```python
from build123d import *

# Parameters (mm, degrees)
F0_W      = 63.5
F0_H      = 50.8
F1_DEPTH  = 88.9
F2_W      = 63.5
F2_H      = 38.1
F3_DEPTH  = 63.501
F5_DEPTH  = 12.701
F7_DEPTH  = 3.048
F9_DEPTH  = 25.401
F11_DEPTH = 50.801


with BuildPart() as f1:
    # F0 (on Front) → F1 (new body)
    with BuildSketch(Plane.XZ):
        Rectangle(F0_W, F0_H)
    extrude(amount=F1_DEPTH)

    # F2 (on face) → F3 (cut, through all)
    with BuildSketch(Plane.YZ.offset(31.75)):
        with Locations((-57.15, 6.35)):
            Rectangle(F2_W, F2_H)
    extrude(amount=-F3_DEPTH, mode=Mode.SUBTRACT)

    # F4 (on face) → F5 (cut, through all)
    with BuildSketch(Plane.XY.offset(-12.7)):
        with BuildLine():
            Line((0, -88.9), (9.5206265251, -88.9))
            Line((9.5206265251, -88.9), (9.5206265251, -57.4386097176))
            ThreePointArc((9.5206265251, -57.4386097176), (0.4771367105, -47.6369581332), (-9.5017243728, -56.4845235209))
            Line((-9.5017243728, -56.4845235209), (-9.5017243728, -88.9))
            Line((-9.5017243728, -88.9), (0, -88.9))
        make_face()
    extrude(amount=-F5_DEPTH, mode=Mode.SUBTRACT)

    # F6 (on face) → F7 (join)
    with BuildSketch(Plane.XY.offset(-12.7)):
        with BuildLine():
            Line((15.748, -88.9), (15.748, -57.15))
            ThreePointArc((15.748, -57.15), (0, -41.402), (-15.748, -57.15))
            Line((-15.748, -57.15), (-15.748, -88.9))
            Line((-15.748, -88.9), (-9.5017243728, -88.9))
            Line((-9.5017243728, -88.9), (-9.5017243728, -56.4845235209))
            ThreePointArc((-9.5017243728, -56.4845235209), (0.4771367105, -47.6369581332), (9.5206265251, -57.4386097176))
            Line((9.5206265251, -57.4386097176), (9.5206265251, -88.9))
            Line((9.5206265251, -88.9), (15.748, -88.9))
        make_face()
    extrude(amount=F7_DEPTH)

    # F8 (on face) → F9 (cut, through all)
    with BuildSketch(Plane.XZ.offset(25.4)):
        with BuildLine():
            ThreePointArc((6.3459234426, 12.927498704), (4.4089615121, 17.2698532126), (0, 19.05))
            Line((0, 19.05), (0, 12.7))
            Line((0, 12.7), (-6.35, 12.7))
            Line((-6.35, 12.7), (-6.35, 0))
            ThreePointArc((-6.35, 0), (0, -6.35), (6.35, 0))
            ThreePointArc((6.35, 0), (6.3499999211, 0.001001282), (6.3499996842, 0.002002564))
            Line((6.3499996842, 0.002002564), (6.3459234426, 12.927498704))
        make_face()
        with BuildLine():
            Line((0, 12.7), (0, 19.05))
            ThreePointArc((0, 19.05), (-4.4901280605, 17.1901280605), (-6.35, 12.7))
            Line((-6.35, 12.7), (0, 12.7))
        make_face()
    extrude(amount=-F9_DEPTH, mode=Mode.SUBTRACT)

    # F10 (on face) → F11 (cut, through all)
    with BuildSketch(Plane.XY.offset(25.4)):
        Polygon((0, -12.7), (0, 0), (-15.24, 0), (-22.352, -12.7), align=None)
        Polygon((15.24, 0), (0, 0), (0, -12.7), (22.352, -12.7), align=None)
    extrude(amount=-F11_DEPTH, mode=Mode.SUBTRACT)


solid = f1.part
```
Check sheet for the modelled part. Datum: model origin and axes. Units: mm. A direction names the side the tool comes from. Coordinates: 2 decimals unless noted, no trailing zeros. Write each loop counter-clockwise with the first axis right and the second up, starting at its lowest first coordinate (ties: lowest second). Pieces come first, ordered by that corner, then holes. Notation, with made-up numbers: (-10.75, 44.25) -> (46.25, 44.25) arc R24 ccw to (46.25, 67.25) -> close; hole circle Ø6 at (16, -39.75). An arc over 180 degrees is marked (long way). Use a Markdown table: item, result.
1. Tool access check on faces 5 (the flat face through (15.748, -73, -11)), 6 (the flat face through (-9.502, -73, -18)), 7 (the flat face through (20, -88.9, -19)), 8 (the cylindrical face through (0.346, -41.406, -11.197)), 9 (the flat face through (-5, -12.7, -5)). Record the directions out of +Z, -Z, +X, -X, +Y, -Y that give a thin tool (end or side, any length) a straight path to the whole face; none if there is none.
Reported:
| item | result |
|---|---|
| face 5 | +Z, +X, -Y |
| face 6 | +Z, -Z, -Y |
| face 7 | +Z, -Z, +X, -X, -Y |
| face 8 | +Z |
| face 9 | +Z, -Z |
2. Release check for a two-part mould opening along Z. For faces 1 (the flat face through (10, -65, -9.652)), 2 (the flat face through (-15.748, -73, -11)), 3 (the flat face through (0, -44, -25.4)), 4 (the cylindrical face through (-0.14, -19.14, -6.35)) record: pulls with the +Z half, pulls with the -Z half, needs draft (parallel to the pull), parting line crosses it, or undercut.
Reported:
| item | result |
|---|---|
| face 1 | pulls with the +Z half |
| face 2 | needs draft |
| face 3 | pulls with the -Z half |
| face 4 | undercut |
3. Sectioned sample at A-A (y = -6.5). Enter the section's corners in (x, z), plus the area to 3 significant figures.
Reported:
| item | result |
|---|---|
| outline | (-31.75, -25.4) -> (-18.88, -25.4) -> (-18.88, 25.4) -> (-31.75, 25.4) -> close; (18.88, -25.4) -> (31.75, -25.4) -> (31.75, 25.4) -> (18.88, 25.4) -> close |
| area | 1,310 mm2 |
4. Go/stop test with flat-tipped pins: pin 1 Ø2.5 at (y, z) = (-78.5, -10.5) entering from -X; pin 2 Ø11.5 at (x, z) = (4, -2) entering from -Y; pin 3 Ø6 at (x, y) = (-22, -43.5) entering from +Z; pin 4 Ø10 at (y, z) = (-34.5, -2.5) entering from -X. Record where each tip stops, or that it passes through.
Reported:
| item | result |
|---|---|
| pin 1 | stops at x = -15.75 |
| pin 2 | stops at y = -25.4 |
| pin 3 | stops at z = -12.7 |
| pin 4 | passes through |
5. Scan lines: line 1 along Z through (x, y) = (-18.5, -48); line 2 along Z through (x, y) = (-5, -24); line 3 along Y through (x, z) = (3.5, -10). Record each from-to range of solid material in increasing order.
Reported:
| item | result |
|---|---|
| line 1 | z = -25.4 to -12.7 |
| line 2 | z = -25.4 to -3.91, 16.61 to 25.4 |
| line 3 | y = -48.29 to -41.8, -25.4 to -12.7 |
6. Sectioned sample at B-B (x = 5). Enter the section's corners in (y, z), plus the area to 3 significant figures.
Reported:
| item | result |
|---|---|
| outline | (-49.04, -25.4) -> (-12.7, -25.4) -> (-12.7, -3.91) -> (-25.4, -3.91) -> (-25.4, -12.7) -> (-42.22, -12.7) -> (-42.22, -9.65) -> (-49.04, -9.65) -> close; (-25.4, 16.61) -> (-12.7, 16.61) -> (-12.7, 25.4) -> (-25.4, 25.4) -> close |
| area | 706 mm2 |
7. Sectioned sample at C-C (z = 10). Enter the section's corners in (x, y), plus the area to 3 significant figures.
Reported:
| item | result |
|---|---|
| outline | (-31.75, -25.4) -> (-6.35, -25.4) -> (-6.35, -12.7) -> (-22.35, -12.7) -> (-15.24, 0) -> (-31.75, 0) -> close; (6.35, -25.4) -> (31.75, -25.4) -> (31.75, 0) -> (15.24, 0) -> (22.35, -12.7) -> (6.35, -12.7) -> close |
| area | 974 mm2 |
8. Sectioned sample at D-D (z = -8). Enter the section's corners in (x, y).
Reported:
| item | result |
|---|---|
| outline | (-31.75, -25.4) -> (31.75, -25.4) -> (31.75, 0) -> (15.24, 0) -> (22.35, -12.7) -> (-22.35, -12.7) -> (-15.24, 0) -> (-31.75, 0) -> close |
